Could you check a few things on this drawing? It's one solid part, dimensions in mm from its lowest x, y, z. Give positions to 0.01 mm unless a question says otherwise; leave off trailing zeros. Loops run counter-clockwise (first coordinate to the right, second up) from the corner with the lowest first, then second, coordinate; pieces in that order, holes last. Notation, with made-up numbers: (19.25, -14.75) - (41.25, -14.75) arc R33 ccw to (41.25, 20.25) - close; hole circle Ø2 at (76.5, 77). An arc over 180 degrees is marked (long way). Use a Markdown table: item, result.
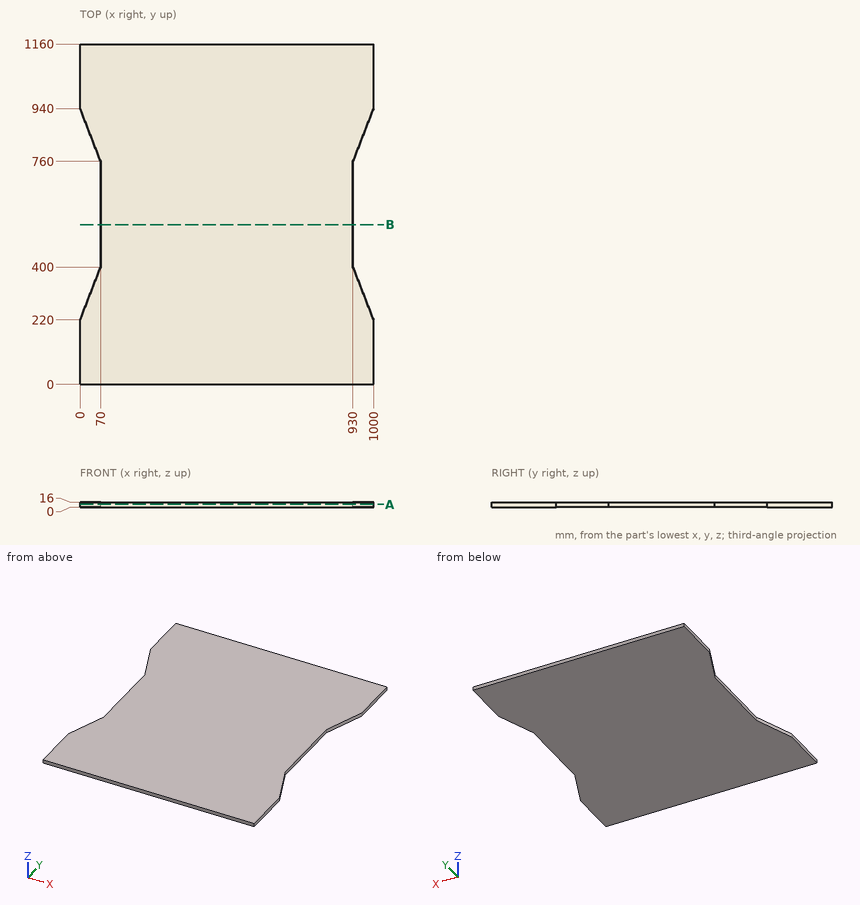
(1) Will these pins go through, and if not, where does the flat tip stop? pin 1 (8 mm diameter, centred on y = 643, z = 8, fed in from +X); pin 2 (1 mm diameter, centred on y = 591.5, z = 5, fed in from -X).
A:
| item | result |
|---|---|
| pin 1 | x = 930 |
| pin 2 | x = 70 |
(2) Suppose I cut it at A-A on z = 9.25. Write out the boundary of the cut face in (x, y).
A:
| item | result |
|---|---|
| outline | (0, 0) - (1000, 0) - (1000, 220) - (930, 400) - (930, 760) - (1000, 940) - (1000, 1160) - (0, 1160) - (0, 940) - (70, 760) - (70, 400) - (0, 220) - close |
(3) If I drill on line 1 (X direction, y = 645, z = 11.5); line 2 (X direction, y = 867.5, z = 8.5), over which ranges is the centre line in solid material (lowest first)?
A:
| item | result |
|---|---|
| line 1 | 70 to 930 |
| line 2 | 28.19 to 971.81 |
(4) Suppose I cut it at B-B on y = 544.5. Write out the boundary of the cut face in (x, z).
A:
| item | result |
|---|---|
| outline | (70, 0) - (930, 0) - (930, 16) - (70, 16) - close |
